Geometry: final body of the model. Coordinates: model frame, mm. A direction names the side the tool comes from. Coordinates: 2 decimals unless noted, no trailing zeros. Write each loop counter-clockwise with the first axis right and the second up, starting at its lowest first coordinate (ties: lowest second). Pieces come first, ordered by that corner, then holes. Notation, with made-up numbers: (33, 69) - (40, 69) arc R20 cw to (40, 95) - close; hole circle Ø4 at (67, 2). An arc over 180 degrees is marked (long way). Answer as a JSON object with one key per item and string values. Group by question number.
Item 1: First-contact query: pin 1 Ø2 at (y, z) = (5, -14.5) entering from +X; pin 2 Ø6 at (x, z) = (-22, -5) entering from +Y. Flat tips, straight axial feed; report the tip coordinate or a pass-through.
Item 2: Set-up query: faces 1 (the flat face through (-13.49, -0.5, -9.4)), 2 (the flat face through (-33.49, 5, -9)). Return all of +Z, -Z, +X, -X, +Y, -Y with unobstructed straight access to the full face (end or side cutting, diameter ignored); none if empty.
Item 3: Section B-B on x = -26.25. Return loops of the section in (y, z), and give its area (3 significant figures).
Item 4: Section C-C on y = 5. Return loops of the section in (x, z).
Item 5: Section A-A on z = -17. Return loops of the section in (x, y), and give its area (3 significant figures).
Item 6: Line query: line 1 along Y through (x, z) = (-19.25, -3.75); line 2 along X through (y, z) = (0.25, -2.25). Output: solid intervals per line, ascending. Write a range as from..to.
```python
from build123d import *

# Parameters (mm, degrees)
BOSS_EXTRUDE1_DEPTH = 10
SKETCH2_W           = 23
SKETCH2_H           = 23
BOSS_EXTRUDE2_DEPTH = 1


with BuildPart() as part:
    # Sketch1 → Boss-Extrude1 (new body)
    with BuildSketch(Plane(origin=(0, 0, 0), x_dir=(1, 0, 0), z_dir=(0, 1, 0))):
        Polygon((-36.489872914, 17.750117647), (-36.489872914, -2.249882353), (-33.489872914, -2.249882353), (-33.489872914, 0.750117647), (-33.489872914, 20.750117647), (-36.489872914, 20.750117647), align=None)
    extrude(amount=BOSS_EXTRUDE1_DEPTH)

    # Sketch2 → Boss-Extrude2 (add)
    with BuildSketch(Plane.XZ):
        with Locations((-24.989872914, -9.250117647)):
            Rectangle(SKETCH2_W, SKETCH2_H)
    extrude(amount=BOSS_EXTRUDE2_DEPTH)


solid = part.part
```
Checks:
{
 "1": {"pin 1": "x = -33.49", "pin 2": "y = 0"},
 "2": {"face 1": "+Z, -Z, +X, +Y, -Y", "face 2": "+Z, -Z, +X, +Y"},
 "3": {"outline": "(-1, -20.75) - (0, -20.75) - (0, 2.25) - (-1, 2.25) - close", "area": "23.0 mm^2"},
 "4": {"outline": "(-36.49, -20.75) - (-33.49, -20.75) - (-33.49, 2.25) - (-36.49, 2.25) - close"},
 "5": {"outline": "(-36.49, -1) - (-13.49, -1) - (-13.49, 0) - (-33.49, 0) - (-33.49, 10) - (-36.49, 10) - close", "area": "53.0 mm^2"},
 "6": {"line 1": "-1..0", "line 2": "-36.49..-33.49"}
}
